from build123d import *

# Parameters (mm, degrees)
SKETCH1_W             = 85
SKETCH1_H             = 30
TOP_SURFACE_DEPTH     = 10
SKETCH6_W             = 25
SKETCH6_H             = 5
TOP_SURFACE_CUT_DEPTH = 91.691785736
SKETCH16_R            = 0.64
BOSS_EXTRUDE14_DEPTH  = 1.3
LPATTERN3_COUNT       = 2
LPATTERN3_PITCH       = 83.7


with BuildPart() as part:
    # Sketch1 → Top surface (new body)
    with BuildSketch(Plane(origin=(0, 0, 0), x_dir=(1, 0, 0), z_dir=(0, 1, 0))):
        with Locations((42.5, 15)):
            Rectangle(SKETCH1_W, SKETCH1_H)
    extrude(amount=TOP_SURFACE_DEPTH)

    # Sketch6 → Top surface cut (cut, through all)
    with BuildSketch(Plane.ZY):
        with Locations((-12.5, 2.5)):
            Rectangle(SKETCH6_W, SKETCH6_H)
    extrude(amount=-TOP_SURFACE_CUT_DEPTH, mode=Mode.SUBTRACT)

    # Sketch16 → Boss-Extrude14 (add)
    with BuildSketch(Plane.ZY):
        with BuildLine():
            Line((0, 10), (0, 5))
            Line((0, 5), (0.51, 5))
            ThreePointArc((0.51, 5), (4.675340546, 3.274659454), (2.95, 7.44))
            Line((2.95, 7.44), (0, 10))
        make_face()
        with Locations((2.95, 5)):
            Circle(SKETCH16_R, mode=Mode.SUBTRACT)
    boss_extrude14 = extrude(amount=-BOSS_EXTRUDE14_DEPTH)

    # LPattern3: Boss-Extrude14 ×2
    with Locations(*[(i * LPATTERN3_PITCH, 0, 0) for i in range(1, LPATTERN3_COUNT)]):
        add(boss_extrude14)


solid = part.part
For this review, take the finished solid that the model builds, in its own axes (mm). A direction names the side the tool comes from. Give positions to 0.01 mm unless a question says otherwise; leave off trailing zeros. Loops run counter-clockwise (first coordinate to the right, second up) from the corner with the lowest first, then second, coordinate; pieces in that order, holes last. Notation, with made-up numbers: M 46.25,80 L 105.25,80 A24 cw 105.25,108 Z; hole C -9.75,19 d7. An arc over 180 degrees is marked long. Put each result on its own line as item: value. Start each with the question number.
(1) Add section B-B, the plane x = 48.5. Write out the cut boundary in (y, z).
(2) Add section A-A, the plane y = 1.25. Write out the cut boundary in (x, z).
(3) Machinability: for faces 4 (the flat face through (42, 0, -28)), 5 (the flat face through (42, 7, 0)), which of the approach directions +Z, -Z, +X, -X, +Y, -Y give a long, thin tool a straight path to every point of the face, cutting with its end or side? Answer none if there is none.
(4) Wall thickness on L1, parallel to X at y = 6, z = 3.5; L2, parallel to Z at x = 59, y = 4.25; L3, parallel to Y at x = 79.5, z = -17.5: over which ranges is each line inside the solid? List them lowest first.
(5) For pin 1 (5.5 mm diameter, centred on x = 47.5, y = 2.5, fed in from +Z); pin 2 (4 mm diameter, centred on x = 27.5, z = -19.5, fed in from -Y); pin 3 (1 mm diameter, centred on y = 5, z = 2.95, fed in from -X), all flat-tipped, find the tip position at first contact; note any pin that passes through.
(6) The part is to be moulded in two halves that separate along X. For faces 1 (the flat face through (42, 5, -30)), 2 (the flat face through (0, 6, -13)), 3 (the flat face through (1.3, 6, 2)), say which applies: +X half, -X half, draft (parallel to the pull), parting line (faces both ways), or undercut.
(7) Add section C-C, the plane z = -18.5. Write out the cut boundary in (x, y), then the cut area to 3 significant figures.
Result:
1. outline: M 0,-30 L 10,-30 L 10,0 L 5,0 L 5,-25 L 0,-25 Z
2. outline: M 0,-30 L 85,-30 L 85,-25 L 0,-25 Z
3. face 4: +Z, -Z, +X, -X, -Y
3. face 5: +Z, +Y, -Y
4. L1: x = 0 to 1.3, 83.7 to 85
4. L2: z = -30 to -25
4. L3: y = 5 to 10
5. pin 1: stops at z = 0
5. pin 2: stops at y = 5
5. pin 3: passes through
6. face 1: draft
6. face 2: -X half
6. face 3: undercut
7. outline: M 0,5 L 85,5 L 85,10 L 0,10 Z
7. area: 425 mm^2
